Part model, mm, in its own coordinate system. Give positions to 0.01 mm unless a question says otherwise; leave off trailing zeros. Write each loop counter-clockwise with the first axis right and the second up, starting at its lowest first coordinate (ties: lowest second). Pieces come first, ordered by that corner, then holes. Notation, with made-up numbers: M -13,81 L 0,81 A25 cw 0,107 Z; hole C 39.5,59.5 d1. An arc over 180 degrees is marked long. Answer as CSV lines item,"result". Start each with the question number.
Item 1: Band-saw the part on D-D, the plane x = 13. List the corners of the cut face in (y, z), then the cut area to 3 significant figures.
Item 2: Band-saw the part on A-A, the plane y = 10.2. List the corners of the cut face in (x, z).
Item 3: Band-saw the part on C-C, the plane x = 7.25. List the corners of the cut face in (y, z), then the cut area to 3 significant figures.
Item 4: Two-plate mould, pull along X, no slides. Class faces 1 (the flat face through (8, 0, 5)), 2 (the cylindrical face through (7.512, 8.004, 5.07)), 3 (the cylindrical face through (13.594, 17.719, 5.07)): +X half, -X half, draft (parallel to the pull), parting line (faces both ways), or undercut.
Item 5: Wall check: L1, parallel to Y at x = 8, z = 9.75; L2, parallel to X at y = 9.5, z = 4.5; L3, parallel to Y at x = 9.75, z = 3.75. Give the ranges that are in metal, low to high. Write a range as from..to.
Item 6: Pin check, flat tips, straight feed: pin 1 (1 mm diameter, centred on y = 14, z = 2.5, fed in from +X); pin 2 (1.5 mm diameter, centred on y = 15, z = 5, fed in from +X). Stop position of each tip, or through.
from build123d import *

# Parameters (mm, degrees)
SKETCH1_W           = 16
SKETCH1_H           = 20
BOSS_EXTRUDE1_DEPTH = 10
SKETCH2_R           = 2.25
CUT_EXTRUDE1_DEPTH  = 28.49545417
FILLET1_R           = 8


with BuildPart() as part:
    # Sketch1 → Boss-Extrude1 (new body)
    with BuildSketch(Plane.XY):
        with Locations((8, 10)):
            Rectangle(SKETCH1_W, SKETCH1_H)
    extrude(amount=BOSS_EXTRUDE1_DEPTH)

    # Sketch2 → Cut-Extrude1 (cut, through all)
    with BuildSketch(Plane.XY.offset(10)):
        with Locations((8, 10.2)):
            Circle(SKETCH2_R)
    extrude(amount=-CUT_EXTRUDE1_DEPTH, mode=Mode.SUBTRACT)

    # Fillet1
    fillet1_edges = [part.edges().sort_by_distance(p)[0] for p in [
        (16, 20, 5),
        (0, 20, 5),
    ]]
    fillet(fillet1_edges, radius=FILLET1_R - 0.0001)  # a hair under: the kernel refuses the full size


solid = part.part
Output:
1,outline,"M 0,0 L 18.25,0 L 18.25,10 L 0,10 Z"
1,area,"182 mm²"
2,outline,"M 0,0 L 5.75,0 L 5.75,10 L 0,10 Z; M 10.25,0 L 16,0 L 16,10 L 10.25,10 Z"
3,outline,"M 0,0 L 8.08,0 L 8.08,10 L 0,10 Z; M 12.32,0 L 19.96,0 L 19.96,10 L 12.32,10 Z"
3,area,"157 mm²"
4,face 1,"draft"
4,face 2,"undercut"
4,face 3,"+X half"
5,L1,"0..7.95, 12.45..20"
5,L2,"0..5.86, 10.14..16"
5,L3,"0..8.79, 11.61..19.81"
6,pin 1,"x = 15.86"
6,pin 2,"x = 15.68"
